The model under review builds one solid part; all positions refer to its coordinate system, in mm. Coordinates: 2 decimals unless noted, no trailing zeros. Order: outer loops, then holes, each group sorted by start corner. A loop starts at its lowest first (then second) coordinate and runs counter-clockwise, first axis right, second up. Notation, with made-up numbers: M -39.75,60 L -12.75,60 A25 ccw -12.75,78 Z; hole C 49,-21.5 d6. An arc over 180 degrees is marked long. Answer in a Markdown table with one row per item.
from build123d import *

# Parameters (mm, degrees)
SKETCH1_R           = 63.737542135
SKETCH1_R_2         = 1.4
BOSS_EXTRUDE1_DEPTH = 10
FILLET1_R           = 2
FILLET2_R           = 2


with BuildPart() as part:
    # Sketch1 → Boss-Extrude1 (new body)
    with BuildSketch(Plane(origin=(0, 0, 0), x_dir=(1, 0, 0), z_dir=(0, 1, 0))):
        with Locations(Location((0, 0, 0), (0, 0, 270))):
            Circle(SKETCH1_R)
        with Locations(Location((20, 15.2, 0), (0, 0, 270))):
            Circle(SKETCH1_R_2, mode=Mode.SUBTRACT)
        with Locations(Location((20, -15.2, 0), (0, 0, 270))):
            Circle(SKETCH1_R_2, mode=Mode.SUBTRACT)
        with Locations(Location((-20, -15.2, 0), (0, 0, 90))):
            Circle(SKETCH1_R_2, mode=Mode.SUBTRACT)
        with Locations(Location((-20, 15.2, 0), (0, 0, 90))):
            Circle(SKETCH1_R_2, mode=Mode.SUBTRACT)
    extrude(amount=BOSS_EXTRUDE1_DEPTH)

    # Fillet1
    fillet1_edges = [part.edges().sort_by_distance(p)[0] for p in [
        (0, 0, -63.737542135),
    ]]
    fillet(fillet1_edges, radius=FILLET1_R)

    # Fillet2
    fillet2_edges = [part.edges().sort_by_distance(p)[0] for p in [
        (0, 10, -63.737542135),
    ]]
    fillet(fillet2_edges, radius=FILLET2_R)


solid = part.part
(1) The part is to be moulded in two halves that separate along Z. For faces 1 (the cylindrical face through (63.195, 4.958, -8.297)), 2 (the cylindrical face through (-19.15, 4.93, -14.09)), 3 (the flat face through (1, 0, -1)), say which applies: +Z half, -Z half, draft (parallel to the pull), parting line (faces both ways), or undercut.
Report:
| item | result |
|---|---|
| face 1 | parting line |
| face 2 | undercut |
| face 3 | draft |
(2) Take a section at A-A (y = 5.25). Write out the cut boundary in (x, z).
Report:
| item | result |
|---|---|
| outline | C 0,0 d127.48; hole C -20,-15.2 d2.8; hole C -20,15.2 d2.8; hole C 20,-15.2 d2.8; hole C 20,15.2 d2.8 |
(3) Insertion check: P1, Ø6, axis at y = 7, z = 42.5, coming from the -X side; P2, Ø1.5, axis at y = 3, z = 36.5, coming from the +X side; P3, Ø6, axis at y = 6, z = 4, coming from the +X side. Each pin has a flat end and moves straight along its axis. Give the tip position at first contact, or say it passes through.
Report:
| item | result |
|---|---|
| P1 | x = -50.02 |
| P2 | x = 52.77 |
| P3 | x = 63.73 |
(4) To check wall thickness, follow line 1 (Z direction, x = -20, y = 6); line 2 (X direction, y = 6, z = 15.2); line 3 (X direction, y = 4.5, z = 37.5). State the ranges of each line that lie inside material, in increasing order. Write a range as [from, to].
Report:
| item | result |
|---|---|
| line 1 | [-60.52, -16.6], [-13.8, 13.8], [16.6, 60.52] |
| line 2 | [-61.9, -21.4], [-18.6, 18.6], [21.4, 61.9] |
| line 3 | [-51.54, 51.54] |
